Source: CAD feature listing. Evaluate the final solid. Frame: model axes, mm. Face numbers are marked on the shaded views. A direction names the side the tool comes from. Give positions to 0.01 mm unless a question says otherwise; leave off trailing zeros. Order: outer loops, then holes, each group sorted by start corner. A loop starts at its lowest first (then second) coordinate and runs counter-clockwise, first axis right, second up.
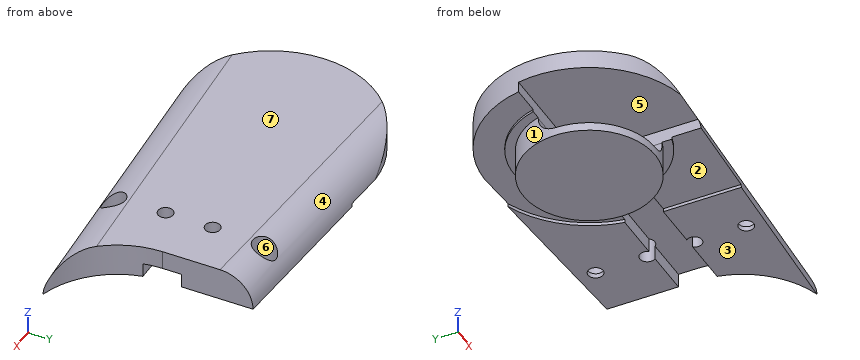
from build123d import *

# Parameters (mm, degrees)
BOSS_EXTRUDE1_DEPTH = 3.5
SKETCH8_R           = 11.5
JOINT_HOLE_DEPTH    = 0.35
JOINT_START         = 0.35
SKETCH3_R           = 7
JOINT_INSERT_DEPTH  = 3.25
FRICTION_START      = 0.35
SKETCH4_R           = 8
SKETCH4_R_2         = 7
FRICTION_DEPTH      = 0.25
CUT_EXTRUDE2_DEPTH  = 43
CUT_EXTRUDE3_DEPTH  = 11
SKETCH2_R           = 0.8
SCREW_HOLES_DEPTH   = 45.522466239
FILLET1_R           = 3.5
CUT_EXTRUDE4_START  = 3.5
SKETCH9_R           = 1.25
CUT_EXTRUDE4_DEPTH  = 3


with BuildPart() as part:
    # Sketch1 → Boss-Extrude1 (new body)
    with BuildSketch(Plane.XY):
        with BuildLine():
            ThreePointArc((-2.526427532, -9.157901721), (-7.558143342, -5.755386106), (-9.5, 0))
            Line((-9.5, 0), (-9.5, 9.59375))
            Line((-9.5, 9.59375), (-32, 11))
            ThreePointArc((-32, 11), (-43, 0), (-32, -11))
            Line((-32, -11), (-2.526427532, -9.157901721))
        make_face()
    extrude(amount=BOSS_EXTRUDE1_DEPTH)

    # Sketch8 → Joint Hole (cut)
    with BuildSketch(Plane.XY):
        with Locations((-32, 0)):
            Circle(SKETCH8_R)
        with BuildLine():
            Line((-20.5, -11.5), (-20.5, 0))
            ThreePointArc((-20.5, 0), (-23.868272016, -8.131727984), (-32, -11.5))
            Line((-32, -11.5), (-20.5, -11.5))
        make_face()
    extrude(amount=JOINT_HOLE_DEPTH, mode=Mode.SUBTRACT)

    # Sketch3 → Joint Insert (add)
    with BuildSketch(Plane.XY.offset(JOINT_START)):
        with Locations((-32, 0)):
            Circle(SKETCH3_R)
    extrude(amount=-JOINT_INSERT_DEPTH)

    # Sketch4 → Friction (add)
    with BuildSketch(Plane.XY.offset(FRICTION_START)):
        with Locations((-32, 0)):
            Circle(SKETCH4_R)
        with Locations((-32, 0)):
            Circle(SKETCH4_R_2, mode=Mode.SUBTRACT)
    extrude(amount=-FRICTION_DEPTH)

    # Sketch6 → Cut-Extrude2 (cut)
    with BuildSketch(Plane(origin=(0, 0, 0), x_dir=(0, 0, -1), z_dir=(1, 0, 0))):
        with BuildLine():
            Line((-1.5, 0), (-1.5, 2))
            Line((-1.5, 2), (0, 2))
            ThreePointArc((0, 2), (2, 0), (0, -2))
            Line((0, -2), (-1.5, -2))
            Line((-1.5, -2), (-1.5, 0))
        make_face()
    extrude(amount=-CUT_EXTRUDE2_DEPTH, mode=Mode.SUBTRACT)

    # Sketch7 → Cut-Extrude3 (cut)
    with BuildSketch(Plane(origin=(0, 0, 0), x_dir=(1, 0, 0), z_dir=(0, 1, 0))):
        with BuildLine():
            Line((-32, -1.5), (-30, -1.5))
            Line((-30, -1.5), (-30, 0))
            ThreePointArc((-30, 0), (-30.585786438, 1.414213562), (-32, 2))
            Line((-32, 2), (-43, 2))
            Line((-43, 2), (-43, -1.5))
            Line((-43, -1.5), (-32, -1.5))
        make_face()
    extrude(amount=-CUT_EXTRUDE3_DEPTH, mode=Mode.SUBTRACT)

    # Sketch2 → Screw Holes (cut, through all)
    with BuildSketch(Plane.XY):
        with Locations((-15, 8)):
            Circle(SKETCH2_R)
        with Locations((-15, -8)):
            Circle(SKETCH2_R)
        with Locations(Location((-15, 2.5, 0), (0, 0, 218.682187453))):
            Circle(SKETCH2_R)
        with Locations(Location((-15, -2.5, 0), (0, 0, 141.317812547))):
            Circle(SKETCH2_R)
    extrude(amount=SCREW_HOLES_DEPTH, mode=Mode.SUBTRACT)

    # Fillet1
    # the kernel refuses this fillet: 3.5 mm, written as the material it takes off along each edge
    with BuildSketch(Plane(origin=(-40.732960062, -11.545810004, 3.5), x_dir=(-0.062378286155180485, 0.9980525784828885, 0), z_dir=(0.9980525784828886, 0.06237828615518049, 0))) as fillet1_piece_1:
        with BuildLine():
            CenterArc((FILLET1_R, -FILLET1_R), FILLET1_R, 90, 90)
            Line((0, -FILLET1_R), (0, 0))
            Line((0, 0), (FILLET1_R, 0))
        make_face()
    extrude(amount=47.031081933, mode=Mode.SUBTRACT)
    with BuildSketch(Plane(origin=(-0.767039938, 9.047939996, 3.5), x_dir=(-0.06237828615518047, -0.9980525784828886, 0), z_dir=(-0.9980525784828886, 0.062378286155180464, 0))) as fillet1_piece_2:
        with BuildLine():
            CenterArc((FILLET1_R, -FILLET1_R), FILLET1_R, 90, 90)
            Line((0, -FILLET1_R), (0, 0))
            Line((0, 0), (FILLET1_R, 0))
        make_face()
    extrude(amount=40.043902481, mode=Mode.SUBTRACT)

    # Sketch9 → Cut-Extrude4 (cut)
    with BuildSketch(Plane.XY.offset(CUT_EXTRUDE4_START)):
        with Locations((-15, 8)):
            Circle(SKETCH9_R)
        with Locations((-15, -8)):
            Circle(SKETCH9_R)
    extrude(amount=-CUT_EXTRUDE4_DEPTH, mode=Mode.SUBTRACT)


solid = part.part
1) Ray query, L1, parallel to Y at x = -15, z = 2.2; L2, parallel to Z at x = -33.5, y = -6.75; L3, parallel to Z at x = -20, y = -0.5. Return the intervals inside material, ascending.
Checks:
L1: y = -6.75 to -3.3, -1.7 to 1.7, 3.3 to 6.75
L2: z = -2.9 to -2, 1.5 to 3.5
L3: z = 1.5 to 3.5
2) Reachability of the marked faces 1, 2 and 3 from +Z, -Z, +X, -X, +Y, -Y: full face, straight path, thin tool, end or side. Return the list, or none.
Checks:
face 1: -Z
face 2: -Z, -Y
face 3: -Z, +X, +Y, -Y
3) Section query B-B on z = 2. Output: boundary loops of the cut face in (x, y), and give its area (3 significant figures).
Checks:
outline: (-35.07, -10.56) - (-3.99, -8.62) arc R9.5 cw to (-9.5, 0) - (-9.5, 8.96) - (-35.07, 10.56) arc R11 ccw to start; hole circle Ø2.5 at (-15, -8); hole circle Ø2.5 at (-15, 8); hole circle Ø1.6 at (-15, -2.5); hole circle Ø1.6 at (-15, 2.5)
area: 623 mm2
4) Section query A-A on y = -2.5. Output: boundary loops of the cut face in (x, z).
Checks:
outline: (-42.71, 1.5) - (-30, 1.5) - (-30, 0) arc R2 cw to (-32, -2) - (-38.54, -2) - (-38.54, -2.9) - (-25.46, -2.9) - (-25.46, 0.1) - (-24.4, 0.1) - (-24.4, 0.35) - (-20.5, 0.35) - (-20.5, 0) - (-15.8, 0) - (-15.8, 3.5) - (-42.71, 3.5) - close; (-14.2, 0) - (-9.17, 0) - (-9.17, 3.5) - (-14.2, 3.5) - close
5) First-contact query: pin 1 Ø3 at (y, z) = (2, 1) entering from +X; pin 2 Ø0.8 at (x, y) = (-15, -7.5) entering from +Z; pin 3 Ø3 at (x, z) = (-21, 1.5) entering from +Y. Flat tips, straight axial feed; report the tip coordinate or a pass-through.
Checks:
pin 1: stops at x = -9.5
pin 2: stops at z = 0.5
pin 3: stops at y = 10.36
6) Section query D-D on z = -1.5. Output: boundary loops of the cut face in (x, y).
Checks:
outline: (-38.87, 1.32) - (-25.13, 1.32) arc R7 ccw to start; (-30.68, -6.87) arc R7 ccw to (-25.13, -1.32) - (-30.68, -1.32) - close
7) Section query C-C on y = 3.75. Output: boundary loops of the cut face in (x, z).
Checks:
outline: (-42.34, 0.35) - (-39.07, 0.35) - (-39.07, 0.1) - (-37.91, 0.1) - (-37.91, -2.9) - (-26.09, -2.9) - (-26.09, 0.1) - (-24.93, 0.1) - (-24.93, 0.35) - (-21.13, 0.35) - (-21.13, 0) - (-9.5, 0) - (-9.5, 3.5) - (-42.34, 3.5) - close
8) Pull-direction query (Y, two-part tool) for the marked faces 4, 5, 6 and 7; classes: +Y half, -Y half, draft (parallel to the pull), parting line (faces both ways), or undercut.
Checks:
face 4: +Y half
face 5: undercut
face 6: undercut
face 7: draft
